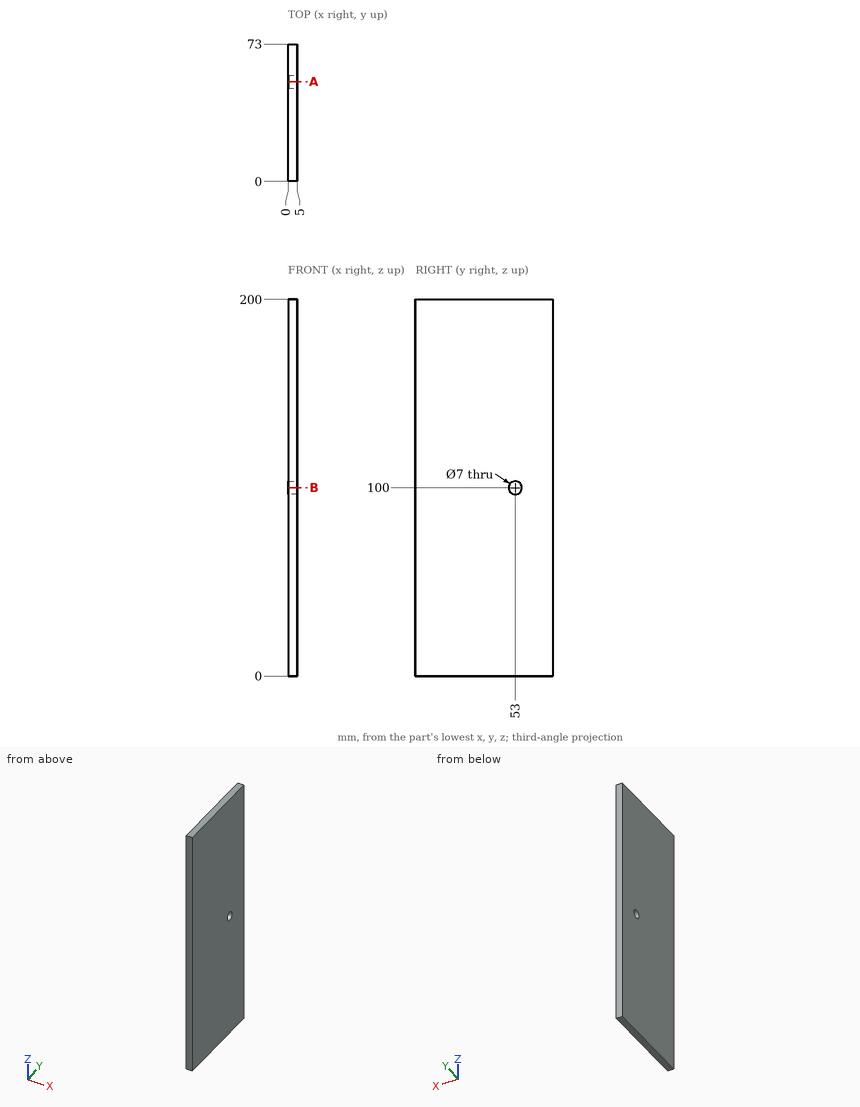
Check sheet for the drawn part. Datum: minimum x, y, z corner. Units: mm. Give positions to 0.01 mm unless a question says otherwise; leave off trailing zeros. Order: outer loops, then holes, each group sorted by start corner. A loop starts at its lowest first (then second) coordinate and runs counter-clockwise, first axis right, second up. Notation, with made-up numbers: (-26.5, 11.5) -> (-14.5, 11.5) arc R32 cw to (-14.5, 49.5) -> close; hole circle Ø2 at (-0.75, 11). An arc over 180 degrees is marked (long way). One line per item, written item: value.
(1) Sectioned sample at A-A on y = 53. Record the cut outline in (x, z), then the cut area to 3 significant figures.
Final values:
outline: (0, 0) -> (5, 0) -> (5, 96.5) -> (0, 96.5) -> close; (0, 103.5) -> (5, 103.5) -> (5, 200) -> (0, 200) -> close
area: 965 mm^2
(2) Sectioned sample at B-B on z = 100. Record the cut outline in (x, y), then the cut area to 3 significant figures.
Final values:
outline: (0, 0) -> (5, 0) -> (5, 49.5) -> (0, 49.5) -> close; (0, 56.5) -> (5, 56.5) -> (5, 73) -> (0, 73) -> close
area: 330 mm^2
(3) Gauge pin test, flat end, axial feed: pin 1 (6.5 mm diameter, centred on y = 53, z = 100, fed in from -X). Record the tip position at first contact, or that the pin passes through.
Final values:
pin 1: through
(4) Scan lines: line 1 along Y through (x, z) = (3.95, 100); line 2 along Z through (x, y) = (1.8, 55.5); line 3 along Z through (x, y) = (1.5, 54.5). Record each from-to range of solid material in increasing order. Write a range as [from, to].
Final values:
line 1: [0, 49.5], [56.5, 73]
line 2: [0, 97.55], [102.45, 200]
line 3: [0, 96.84], [103.16, 200]
